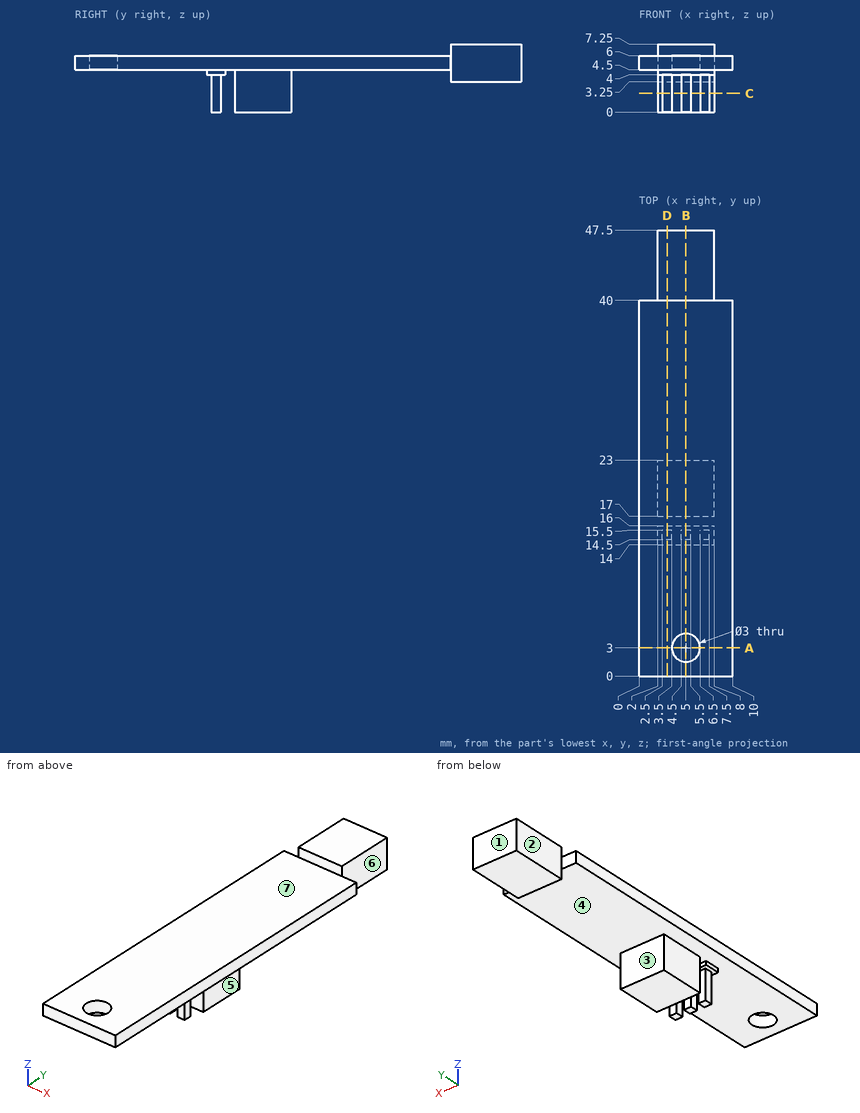
Here's the drawing with two shaded views (mm, measured from the low corner). I have some questions. A direction names the side the tool comes from. Coordinates: 2 decimals unless noted, no trailing zeros. Loops run counter-clockwise (first coordinate to the right, second up) from the corner with the lowest first, then second, coordinate; pieces in that order, holes last. Notation, with made-up numbers: (63.5, -24.75) -> (99.5, -24.75) arc R15 cw to (99.5, 3.25) -> close; hole circle Ø1 at (28, 35.25). An arc over 180 degrees is marked (long way). Use one line per item in the form item = value. Start each with the question number.
(1) On a 3-axis mill with a long thin cutter (end or side, diameter ignored), from which of +Z, -Z, +X, -X, +Y, -Y can I reach the whole of each face in a straight line? I mean the marked faces 5, 6 and 7. Say none if no direction works.
(2) If we section it at B-B (x = 5): Please give me the cut outline in (y, z), then the cut area to 4 significant figures.
(3) Please list where these lines run through material, in increasing order: line 1 along Y through (x, z) = (5, 4.9); line 2 along Y through (x, z) = (3.25, 2.5); line 3 along X through (y, z) = (18, 1).
(4) Will these pins go through, and if not, where does the flat tip stop? pin 1 (2 mm diameter, centred on y = 45.5, z = 5, fed in from -X); pin 2 (1.3 mm diameter, centred on x = 4, z = 3, fed in from -Y); pin 3 (2 mm diameter, centred on x = 4.5, y = 34, fed in from -Z).
(5) If we section it at D-D (x = 3): Please give me the cut outline in (y, z).
(6) If we section it at C-C (z = 2): Please give me the cut outline in (x, y).
(7) If we section it at A-A (y = 3): Please give me the cut outline in (x, z), then the cut area to 3 significant figures.
(8) We'd pull the mould along Y, two halves only. Please class the marked faces 1, 2, 3 and 4: pulls with the +Y half, pulls with the -Y half, needs draft (parallel to the pull), parting line crosses it, or undercut.
Verdict:
q1.face_5 = -Z, +X, +Y, -Y
q1.face_6 = +Z, -Z, +X, +Y
q1.face_7 = +Z, +X, -X, -Y
q2.outline = (0, 4.5) -> (1.5, 4.5) -> (1.5, 6) -> (0, 6) -> close; (4.5, 4.5) -> (14, 4.5) -> (14, 4) -> (14.5, 4) -> (14.5, 0) -> (15.5, 0) -> (15.5, 4) -> (16, 4) -> (16, 4.5) -> (17, 4.5) -> (17, 0) -> (23, 0) -> (23, 4.5) -> (40, 4.5) -> (40, 3.25) -> (47.5, 3.25) -> (47.5, 7.25) -> (40, 7.25) -> (40, 6) -> (4.5, 6) -> close
q2.area = 117.5 mm²
q3.line_1 = 0 to 1.5, 4.5 to 47.5
q3.line_2 = 14.5 to 15.5, 17 to 23
q3.line_3 = 2 to 8
q4.pin_1 = 2
q4.pin_2 = 14.5
q4.pin_3 = 4.5
q5.outline = (0, 4.5) -> (14, 4.5) -> (14, 4) -> (14.5, 4) -> (14.5, 0) -> (15.5, 0) -> (15.5, 4) -> (16, 4) -> (16, 4.5) -> (17, 4.5) -> (17, 0) -> (23, 0) -> (23, 4.5) -> (40, 4.5) -> (40, 3.25) -> (47.5, 3.25) -> (47.5, 7.25) -> (40, 7.25) -> (40, 6) -> (0, 6) -> close
q6.outline = (2, 17) -> (8, 17) -> (8, 23) -> (2, 23) -> close; (2.5, 14.5) -> (3.5, 14.5) -> (3.5, 15.5) -> (2.5, 15.5) -> close; (4.5, 14.5) -> (5.5, 14.5) -> (5.5, 15.5) -> (4.5, 15.5) -> close; (6.5, 14.5) -> (7.5, 14.5) -> (7.5, 15.5) -> (6.5, 15.5) -> close
q7.outline = (0, 4.5) -> (3.5, 4.5) -> (3.5, 6) -> (0, 6) -> close; (6.5, 4.5) -> (10, 4.5) -> (10, 6) -> (6.5, 6) -> close
q7.area = 10.5 mm²
q8.face_1 = pulls with the +Y half
q8.face_2 = needs draft
q8.face_3 = undercut
q8.face_4 = undercut
